The model under review builds one solid part; all positions refer to its coordinate system, in mm. Face numbers are marked on the shaded views. A direction names the side the tool comes from. Round coordinates to 2 decimals unless told otherwise and drop trailing zeros. Write each loop counter-clockwise with the first axis right and the second up, starting at its lowest first coordinate (ties: lowest second). Pieces come first, ordered by that corner, then holes. Notation, with made-up numbers: (-14, 35.5) -> (4, 35.5) arc R28 cw to (4, 64.5) -> close; hole circle Ø5 at (-18.5, 62). An arc over 180 degrees is marked (long way). Return JSON: item names as keys, results as strings. Group by question number.
1. Take a section at A-A, the plane y = 0. Write out the cut boundary in (x, z).
2. Take a section at B-B, the plane x = 0. Write out the cut boundary in (y, z).
3. Take a section at C-C, the plane z = -4. Write out the cut boundary in (x, y).
4. Clearance check with flat-ended pins moving along their axes: P1, Ø0.8, axis at y = 6.5, z = -1.5, coming from the +X side; P2, Ø1, axis at x = -4, y = -5, coming from the -Z side; P3, Ø2, axis at x = 1, z = -59, coming from the +Y side. State where each tip first meets the part, or that it passes through.
5. Take a section at D-D, the plane z = -70. Write out the cut boundary in (x, y), then the cut area to 3 significant figures.
6. For line 1 along Z through (x, y) = (-1, -5); line 2 along X through (y, z) = (-5.75, -12); line 3 along Y through (x, z) = (4.75, -13), list the stretches that pass through material, from the lowest coordinate up. Write a range as from..to.
7. Tool access review of the marked faces 1, 2 and 3: name each direction out of +Z, -Z, +X, -X, +Y, -Y from which nothing blocks a thin tool from reaching the whole face with its end or side.
Autodesk Inventor part; units mm, degrees
ref_plane "Work Plane1" through (0, 0, 14.5) normal (0, 0, 1) x (1, 0, 0)
ref_plane "Work Plane2" through (0, 7, -32) normal (0, 1, 0) x (1, 0, 0)
ref_plane "YZ Plane" through (0, 0, 0) normal (1, 0, 0) x (0, 1, 0)
sketch "Sketch1" plane through (0, 0, 0) normal (1, 0, 0) x (0, 1, 0)
  line L0 (0, 0) -> (7, 0)
  line L1 (7, 0) -> (7, -64)
  line L2 (7, -64) -> (0, -64)
  line L3 (0, 0) -> (0, -64)
  line L4 (0, 18.3308) -> (0, -79.8767)
  line L5 (0, -64) -> (4, -64)
  line L6 (4, -64) -> (4, -76)
  line L7 (4, -76) -> (4, -76)
  line L8 (0, -76) -> (0, -74)
  line L9 (0, -76) -> (4, -76)
  line L10 (0, -74) -> (0, -76)
  line L11 (4, -76) -> (0, -76)
  line L12 (0, -74) -> (0, -64)
  line L13 (0, 0) -> (4, 0)
  line L14 (4, 0) -> (4, 17.5)
  line L15 (4, 17.5) -> (0, 17.5)
  line L16 (0, 17.5) -> (0, 0)
  point P0 (0, -82)
  point P1 (0, -64)
  point P2 (0, 17.5)
  point P3 (4, 0)
  point P4 (0, -76)
  dimension "d0" = 7
  dimension "d1" = 64
  dimension "d7" = 12
  dimension "d11" = 4
  dimension "d35" = 4
  dimension "d36" = 17.5
ref_plane "Work Plane1" through (0, 0, 14.5) normal (0, 0, 1) x (1, 0, 0)
revolve "Revolution2" add sketch "Sketch1" angle 360 about axis through (0, 0, 18.3308) along (0, 0, -1)
sketch "Sketch4" plane through (0, 0, 0) normal (0, 0, 1) x (1, 0, 0)
  line L0 (0, 7) -> (2.5, 7)
  line L1 (2.5, 7) -> (-2.5, 7)
  line L2 (-2.5, 7) -> (-2.5, 5.5)
  line L3 (-2.5, 5.5) -> (2.5, 5.5)
  line L4 (2.5, 5.5) -> (2.5, 7)
  circle A0 centre (0, 0) radius 7
  point P0 (0, 0)
  point P1 (0, 7)
  dimension "d37" = 2.5
  dimension "d38" = 5
  dimension "d39" = 1.5
extrude "Extrusion5" cut sketch "Sketch4" against normal blind 5.5 contours A0 L2 L1 | L0 L4 A0 | A0 L4 L3 L2 picked at (0, 6)
sketch "Sketch5" plane through (0, 0, -64) normal (0, 0, -1) x (-1, 0, 0)
  line L0 (0, 7) -> (2.5, 7)
  line L1 (2.5, 7) -> (-2.5, 7)
  line L2 (-2.5, 7) -> (-2.5, 5.5)
  line L3 (-2.5, 5.5) -> (2.5, 5.5)
  line L4 (2.5, 5.5) -> (2.5, 7)
  circle A0 centre (0, 0) radius 7
  point P0 (0, 0)
  point P1 (0, 7)
  dimension "d42" = 2.5
  dimension "d43" = 5
  dimension "d44" = 1.5
extrude "Extrusion6" cut sketch "Sketch5" against normal blind 5.5 contours A0 L2 L1 | L0 L4 A0 | A0 L4 L3 L2 picked at (0, 6)
ref_plane "Work Plane2" through (0, 7, -32) normal (0, 1, 0) x (1, 0, 0)
sketch "Sketch6" plane through (0, 7, -32) normal (0, 1, 0) x (1, 0, 0)
  line L0 (2.5, -26.5) -> (-2.5, -26.5)
  circle A0 centre (0, -26.5) radius 2.5
  line L1 (-2.5, 26.5) -> (2.5, 26.5)
  circle A1 centre (0, 26.5) radius 2.5
  point P0 (0, -32)
extrude "Extrusion7" cut sketch "Sketch6" against normal blind 1.5
fillet "Fillet4" radius 0.35 6 edges at (0, 5.5, -8) (2.5, 5.5, -2.75) (-2.5, 5.5, -2.75) (-2.5, 5.5, -61.25) (2.5, 5.5, -61.25) (0, 5.5, -56)
fillet "Fillet5" radius 0.5 2 edges at (0, -4, 0) (0, -4, -64)
properties part number "eje1" material "PBT Plastic"
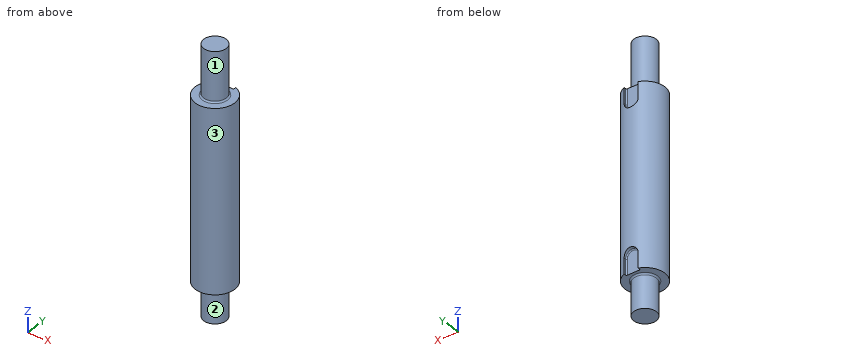
Output:
{
 "1": {"outline": "(-7, -64) -> (-4.5, -64) arc R0.5 cw to (-4, -64.5) -> (-4, -76) -> (4, -76) -> (4, -64.5) arc R0.5 cw to (4.5, -64) -> (7, -64) -> (7, 0) -> (4.5, 0) arc R0.5 cw to (4, 0.5) -> (4, 17.5) -> (-4, 17.5) -> (-4, 0.5) arc R0.5 cw to (-4.5, 0) -> (-7, 0) -> close"},
 "2": {"outline": "(-7, -64) -> (-4.5, -64) arc R0.5 cw to (-4, -64.5) -> (-4, -76) -> (4, -76) -> (4, -64.5) arc R0.5 cw to (4.5, -64) -> (5.5, -64) -> (5.5, -56.35) arc R0.35 cw to (5.85, -56) -> (7, -56) -> (7, -8) -> (5.85, -8) arc R0.35 cw to (5.5, -7.65) -> (5.5, 0) -> (4.5, 0) arc R0.5 cw to (4, 0.5) -> (4, 17.5) -> (-4, 17.5) -> (-4, 0.5) arc R0.5 cw to (-4.5, 0) -> (-7, 0) -> close"},
 "3": {"outline": "(-2.5, 5.85) -> (-2.5, 6.54) arc R7 ccw (long way) to (2.5, 6.54) -> (2.5, 5.85) arc R0.35 cw to (2.15, 5.5) -> (-2.15, 5.5) arc R0.35 cw to start"},
 "4": {"P1": "stops at x = 3.43", "P2": "stops at z = -64", "P3": "stops at y = 5.5"},
 "5": {"outline": "circle Ø8 at (0, 0)", "area": "50.3 mm^2"},
 "6": {"line 1": "z = -64..0", "line 2": "x = -3.99..3.99", "line 3": "y = -5.14..5.14"},
 "7": {"face 1": "+Z", "face 2": "-Z", "face 3": "+Z, -Z"}
}
